Check sheet for the modelled part. Datum: model origin and axes. Units: mm. A direction names the side the tool comes from. Coordinates: 2 decimals unless noted, no trailing zeros. Loops run counter-clockwise (first coordinate to the right, second up) from the corner with the lowest first, then second, coordinate; pieces in that order, holes last. Notation, with made-up numbers: (16, 69.25) - (74, 69.25) arc R28 cw to (74, 98.25) - close; hole circle Ø1 at (-38.75, -5.5). An arc over 180 degrees is marked (long way). Use a Markdown table: item, result. Add a question column.
1) Sectioned sample at B-B, the plane y = 16. Enter the section's corners in (x, z), then the cut area to 3 significant figures.
2) Sectioned sample at C-C, the plane z = 52. Enter the section's corners in (x, y), then the cut area to 3 significant figures.
3) Go/stop test with flat-tipped pins: P1, Ø12, axis at y = 5.5, z = -48, coming from the -X side; P2, Ø6, axis at x = -9, y = -3.5, coming from the -Z side; P3, Ø12, axis at y = -6, z = -45, coming from the +X side; P4, Ø12, axis at y = -3, z = 40.5, coming from the -X side. Record where each tip stops, or that it passes through.
4) Thickness scan on line 1 (Z direction, x = 3.75, y = 0); line 2 (Y direction, x = -2.5, z = -40); line 3 (Z direction, x = -3.5, y = -6.5). Record the ranges inside material, lowest first.
5) Tool access check on faces 4 (the flat face through (15, 0, 20)), 5 (the flat face through (-15, 0, -20)), 6 (the flat face through (10, 0, -27)), 7 (the flat face through (-10, 0, 27)). Record the directions out of +Z, -Z, +X, -X, +Y, -Y that give a thin tool (end or side, any length) a straight path to the whole face; none if there is none.
6) Sectioned sample at A-A, the plane x = 1.5. Enter the section's corners in (y, z).
7) Sectioned sample at D-D, the plane x = -14.5. Enter the section's corners in (y, z), then the cut area to 3 significant figures.
8) Draft check along Z on faces 1 (the flat face through (-15, 0, 20)), 2 (the flat face through (-20, 0, 0)), 3 (the cylindrical face through (-0.14, -2.17, 30.24)). Enter one of: pulls with the +Z half, pulls with the -Z half, needs draft (parallel to the pull), parting line crosses it, or undercut.
from build123d import *

# Parameters (mm, degrees)
F0_R     = 10
F1_DEPTH = 10
F2_W     = 40
F2_H     = 20
F3_DEPTH = 10


with BuildPart() as f1:
    # F0 (on Right) → F1 (new body)
    with BuildSketch(Plane.YZ):
        with BuildLine():
            Line((-20, 40), (-20, 0))
            Line((-20, 0), (20, 0))
            Line((20, 0), (20, 40))
            ThreePointArc((20, 40), (14.142136, 54.142136), (0, 60))
            ThreePointArc((0, 60), (-14.142136, 54.142136), (-20, 40))
        make_face()
        with Locations((0, 40)):
            Circle(F0_R, mode=Mode.SUBTRACT)
    extrude(amount=F1_DEPTH)

    # F2 (on face) → F3 (join)
    with BuildSketch(Plane.YZ.offset(10)):
        with Locations((0, 10)):
            Rectangle(F2_W, F2_H)
    extrude(amount=F3_DEPTH)

    # F4: F1 across plane


with BuildPart() as f1_1:
    add(f1.part)
    add(f1.part.mirror(Plane.YZ))

    # F5: F1 across plane


with BuildPart() as f1_2:
    add(f1_1.part)
    add(f1_1.part.mirror(Plane.XY))


solid = f1_2.part
Solved:
| question | item | result |
|---|---|---|
| 1 | outline | (-20, -20) - (-10, -20) - (-10, -52) - (10, -52) - (10, -20) - (20, -20) - (20, 20) - (10, 20) - (10, 52) - (-10, 52) - (-10, 20) - (-20, 20) - close |
| 1 | area | 2,880 mm2 |
| 2 | outline | (-10, -16) - (10, -16) - (10, 16) - (-10, 16) - close |
| 2 | area | 640 mm2 |
| 3 | P1 | stops at x = -10 |
| 3 | P2 | stops at z = -59.99 |
| 3 | P3 | stops at x = 10 |
| 3 | P4 | passes through |
| 4 | line 1 | z = -60 to -50, -30 to 30, 50 to 60 |
| 4 | line 2 | y = -20 to -10, 10 to 20 |
| 4 | line 3 | z = -58.91 to -47.6, -32.4 to 32.4, 47.6 to 58.91 |
| 5 | face 4 | +Z, +X, +Y, -Y |
| 5 | face 5 | -Z, -X, +Y, -Y |
| 5 | face 6 | -Z, +X, +Y, -Y |
| 5 | face 7 | +Z, -X, +Y, -Y |
| 6 | outline | (-20, -40) arc R20 ccw to (0, -60) arc R20 ccw to (20, -40) - (20, 40) arc R20 ccw to (0, 60) arc R20 ccw to (-20, 40) - close; hole circle Ø20 at (0, -40); hole circle Ø20 at (0, 40) |
| 7 | outline | (-20, -20) - (20, -20) - (20, 20) - (-20, 20) - close |
| 7 | area | 1,600 mm2 |
| 8 | face 1 | pulls with the +Z half |
| 8 | face 2 | needs draft |
| 8 | face 3 | undercut |
